Can you work these out from the model? Positions are in its coordinate system, mm. A direction names the side the tool comes from. Give positions to 0.01 mm unless a question says otherwise; leave off trailing zeros. Loops run counter-clockwise (first coordinate to the right, second up) from the corner with the lowest first, then second, coordinate; pieces in that order, holes last. Notation, with made-up numbers: (8, -15.5) -> (50, -15.5) arc R14 ccw to (50, -9.5) -> close; hole circle Ø7 at (37.5, 6.25). An arc over 180 degrees is marked (long way). Use CSV: the item, a comma, the result in double quotes.
from build123d import *

# Parameters (mm, degrees)
F1_DEPTH = 2
F3_DEPTH = 2
F5_DEPTH = 2


with BuildPart() as f1:
    # F0 (on Top) → F1 (new body)
    with BuildSketch(Plane.XY):
        with BuildLine():
            ThreePointArc((49.942072, -2.406128), (49.985516, -1.203413), (50, 0))
            ThreePointArc((50, 0), (49.974201, 1.606012), (49.896829, 3.210366))
            ThreePointArc((49.896829, 3.210366), (43.993208, 6.785947), (48.544998, 11.974273))
            ThreePointArc((48.544998, 11.974273), (47.87884, 14.408911), (47.090663, 16.806829))
            ThreePointArc((47.090663, 16.806829), (40.967156, 18.934106), (43.314795, 24.976559))
            ThreePointArc((43.314795, 24.976559), (41.843566, 27.369983), (40.240229, 29.676994))
            ThreePointArc((40.240229, 29.676994), (33.340682, 29.493226), (34.36487, 36.318806))
            ThreePointArc((34.36487, 36.318806), (32.488197, 38.006802), (30.528729, 39.597938))
            ThreePointArc((30.528729, 39.597938), (24.227214, 38.076901), (22.935377, 44.429365))
            ThreePointArc((22.935377, 44.429365), (20.403718, 45.647435), (17.80764, 46.721386))
            ThreePointArc((17.80764, 46.721386), (12.102725, 42.836614), (9.274139, 49.132376))
            ThreePointArc((9.274139, 49.132376), (6.782782, 49.537802), (4.274139, 49.816982))
            ThreePointArc((4.274139, 49.816982), (-0.204697, 45.130548), (-4.725861, 49.776161))
            ThreePointArc((-4.725861, 49.776161), (-7.514166, 49.432148), (-10.278748, 48.932069))
            ThreePointArc((-10.278748, 48.932069), (-12.977762, 42.57968), (-18.761065, 46.346763))
            ThreePointArc((-18.761065, 46.346763), (-21.076119, 45.3409), (-23.337459, 44.219487))
            ThreePointArc((-23.337459, 44.219487), (-24.571619, 37.855565), (-30.886672, 39.319378))
            ThreePointArc((-30.886672, 39.319378), (-33.046356, 37.522505), (-35.101707, 35.607165))
            ThreePointArc((-35.101707, 35.607165), (-33.937901, 28.803999), (-40.839764, 28.84638))
            ThreePointArc((-40.839764, 28.84638), (-42.243501, 26.748582), (-43.53958, 24.582616))
            ThreePointArc((-43.53958, 24.582616), (-41.137225, 18.561708), (-47.241183, 16.37897))
            ThreePointArc((-47.241183, 16.37897), (-48.086561, 13.69973), (-48.780121, 10.977238))
            ThreePointArc((-48.780121, 10.977238), (-44.122996, 5.883251), (-49.952127, 2.187476))
            ThreePointArc((-49.952127, 2.187476), (-49.99887, -0.336221), (-49.918191, -2.859061))
            ThreePointArc((-49.918191, -2.859061), (-44.642053, -6.62536), (-48.596952, -11.761645))
            ThreePointArc((-48.596952, -11.761645), (-47.859623, -14.472611), (-46.971192, -17.137885))
            ThreePointArc((-46.971192, -17.137885), (-40.299352, -18.905387), (-43.205042, -25.165937))
            ThreePointArc((-43.205042, -25.165937), (-41.879951, -27.314277), (-40.448129, -29.393007))
            ThreePointArc((-40.448129, -29.393007), (-33.973344, -29.708924), (-34.523532, -36.168021))
            ThreePointArc((-34.523532, -36.168021), (-32.437593, -38.050001), (-30.249241, -39.81185))
            ThreePointArc((-30.249241, -39.81185), (-23.680948, -37.691698), (-22.740661, -44.529342))
            ThreePointArc((-22.740661, -44.529342), (-20.464443, -45.620243), (-18.136072, -46.59488))
            ThreePointArc((-18.136072, -46.59488), (-12.518339, -43.360114), (-9.489135, -49.091306))
            ThreePointArc((-9.489135, -49.091306), (-6.716856, -49.546784), (-3.92337, -49.845834))
            ThreePointArc((-3.92337, -49.845834), (0.455989, -44.511162), (4.943718, -49.754996))
            ThreePointArc((4.943718, -49.754996), (7.44838, -49.442104), (9.934059, -49.003209))
            ThreePointArc((9.934059, -49.003209), (12.91115, -43.244774), (18.557995, -46.428448))
            ThreePointArc((18.557995, -46.428448), (21.136435, -45.312814), (23.648143, -44.054118))
            ThreePointArc((23.648143, -44.054118), (24.448153, -37.198646), (31.058502, -39.18379))
            ThreePointArc((31.058502, -39.18379), (32.996395, -37.566446), (34.850197, -35.853364))
            ThreePointArc((34.850197, -35.853364), (34.241441, -29.399524), (40.713093, -29.024886))
            ThreePointArc((40.713093, -29.024886), (42.279058, -26.692345), (43.711539, -24.275531))
            ThreePointArc((43.711539, -24.275531), (40.678202, -18.075823), (47.312431, -16.172008))
            ThreePointArc((47.312431, -16.172008), (48.068288, -13.763707), (48.701644, -11.32033))
            ThreePointArc((48.701644, -11.32033), (44.700316, -6.220133), (49.942072, -2.406128))
        make_face()
    extrude(amount=F1_DEPTH)

    # F2 (on face) → F3 (cut)
    with BuildSketch(Plane.XY.offset(2)):
        with BuildLine():
            Line((8.49059, 0.399851), (9.988929, 0.470413))
            ThreePointArc((9.988929, 0.470413), (9.727268, 2.319537), (9.126347, 4.087762))
            Line((9.126347, 4.087762), (7.738448, 3.516591))
            ThreePointArc((7.738448, 3.516591), (7.46517, 4.064633), (7.153141, 4.591576))
            Line((7.153141, 4.591576), (8.41546, 5.401854))
            ThreePointArc((8.41546, 5.401854), (7.264293, 6.872412), (5.859767, 8.103279))
            Line((5.859767, 8.103279), (4.943397, 6.914682))
            ThreePointArc((4.943397, 6.914682), (4.43271, 7.25266), (3.899014, 7.552992))
            Line((3.899014, 7.552992), (4.587075, 8.885873))
            ThreePointArc((4.587075, 8.885873), (2.854856, 9.58383), (1.023068, 9.947529))
            Line((1.023068, 9.947529), (0.823767, 8.459989))
            ThreePointArc((0.823767, 8.459989), (0.21251, 8.497343), (-0.399851, 8.49059))
            Line((-0.399851, 8.49059), (-0.470413, 9.988929))
            ThreePointArc((-0.470413, 9.988929), (-2.319537, 9.727268), (-4.087762, 9.126347))
            Line((-4.087762, 9.126347), (-3.516591, 7.738448))
            ThreePointArc((-3.516591, 7.738448), (-4.064633, 7.46517), (-4.591576, 7.153141))
            Line((-4.591576, 7.153141), (-5.401854, 8.41546))
            ThreePointArc((-5.401854, 8.41546), (-6.872412, 7.264293), (-8.103279, 5.859767))
            Line((-8.103279, 5.859767), (-6.914682, 4.943397))
            ThreePointArc((-6.914682, 4.943397), (-7.25266, 4.43271), (-7.552992, 3.899014))
            Line((-7.552992, 3.899014), (-8.885873, 4.587075))
            ThreePointArc((-8.885873, 4.587075), (-9.58383, 2.854856), (-9.947529, 1.023068))
            Line((-9.947529, 1.023068), (-8.459989, 0.823767))
            ThreePointArc((-8.459989, 0.823767), (-8.497343, 0.21251), (-8.49059, -0.399851))
            Line((-8.49059, -0.399851), (-9.988929, -0.470413))
            ThreePointArc((-9.988929, -0.470413), (-9.727268, -2.319537), (-9.126347, -4.087762))
            Line((-9.126347, -4.087762), (-7.738448, -3.516591))
            ThreePointArc((-7.738448, -3.516591), (-7.46517, -4.064633), (-7.153141, -4.591576))
            Line((-7.153141, -4.591576), (-8.41546, -5.401854))
            ThreePointArc((-8.41546, -5.401854), (-7.264293, -6.872412), (-5.859767, -8.103279))
            Line((-5.859767, -8.103279), (-4.943397, -6.914682))
            ThreePointArc((-4.943397, -6.914682), (-4.43271, -7.25266), (-3.899014, -7.552992))
            Line((-3.899014, -7.552992), (-4.587075, -8.885873))
            ThreePointArc((-4.587075, -8.885873), (-2.854856, -9.58383), (-1.023068, -9.947529))
            Line((-1.023068, -9.947529), (-0.823767, -8.459989))
            ThreePointArc((-0.823767, -8.459989), (-0.21251, -8.497343), (0.399851, -8.49059))
            Line((0.399851, -8.49059), (0.470413, -9.988929))
            ThreePointArc((0.470413, -9.988929), (2.319537, -9.727268), (4.087762, -9.126347))
            Line((4.087762, -9.126347), (3.516591, -7.738448))
            ThreePointArc((3.516591, -7.738448), (4.064633, -7.46517), (4.591576, -7.153141))
            Line((4.591576, -7.153141), (5.401854, -8.41546))
            ThreePointArc((5.401854, -8.41546), (6.872412, -7.264293), (8.103279, -5.859767))
            Line((8.103279, -5.859767), (6.914682, -4.943397))
            ThreePointArc((6.914682, -4.943397), (7.25266, -4.43271), (7.552992, -3.899014))
            Line((7.552992, -3.899014), (8.885873, -4.587075))
            ThreePointArc((8.885873, -4.587075), (9.58383, -2.854856), (9.947529, -1.023068))
            Line((9.947529, -1.023068), (8.459989, -0.823767))
            ThreePointArc((8.459989, -0.823767), (8.497343, -0.21251), (8.49059, 0.399851))
        make_face()
    extrude(amount=-F3_DEPTH, mode=Mode.SUBTRACT)

    # F4 (on face) → F5 (cut)
    with BuildSketch(Plane.XY.offset(2)):
        with BuildLine():
            ThreePointArc((18.809128, 25.888544), (25.793139, 26.994703), (24.686981, 33.978714))
            ThreePointArc((24.686981, 33.978714), (12.978714, 39.944374), (0, 42))
            ThreePointArc((0, 42), (3.535534, 40.535534), (5, 37))
            ThreePointArc((5, 37), (3.535534, 33.464466), (0, 32))
            ThreePointArc((0, 32), (9.888544, 30.433809), (18.809128, 25.888544))
        make_face()
        with BuildLine():
            ThreePointArc((5, 37), (3.535534, 40.535534), (0, 42))
            ThreePointArc((0, 42), (-5, 37), (0, 32))
            ThreePointArc((0, 32), (3.535534, 33.464466), (5, 37))
        make_face()
        with BuildLine():
            ThreePointArc((-30.433809, 9.888544), (-25.888544, 18.809128), (-18.809128, 25.888544))
            ThreePointArc((-18.809128, 25.888544), (-17.702969, 32.872555), (-24.686981, 33.978714))
            ThreePointArc((-24.686981, 33.978714), (-33.978714, 24.686981), (-39.944374, 12.978714))
            ThreePointArc((-39.944374, 12.978714), (-36.734176, 6.678346), (-30.433809, 9.888544))
        make_face()
        with BuildLine():
            ThreePointArc((-18.809128, -25.888544), (-25.888544, -18.809128), (-30.433809, -9.888544))
            ThreePointArc((-30.433809, -9.888544), (-36.734176, -6.678346), (-39.944374, -12.978714))
            ThreePointArc((-39.944374, -12.978714), (-33.978714, -24.686981), (-24.686981, -33.978714))
            ThreePointArc((-24.686981, -33.978714), (-17.702969, -32.872555), (-18.809128, -25.888544))
        make_face()
        with BuildLine():
            ThreePointArc((18.809128, -25.888544), (9.888544, -30.433809), (0, -32))
            ThreePointArc((0, -32), (-5, -37), (0, -42))
            ThreePointArc((0, -42), (12.978714, -39.944374), (24.686981, -33.978714))
            ThreePointArc((24.686981, -33.978714), (25.793139, -26.994703), (18.809128, -25.888544))
        make_face()
        with BuildLine():
            ThreePointArc((30.433809, 9.888544), (32, 0), (30.433809, -9.888544))
            ThreePointArc((30.433809, -9.888544), (33.644006, -16.188911), (39.944374, -12.978714))
            ThreePointArc((39.944374, -12.978714), (42, 0), (39.944374, 12.978714))
            ThreePointArc((39.944374, 12.978714), (33.644006, 16.188911), (30.433809, 9.888544))
        make_face()
    extrude(amount=-F5_DEPTH, mode=Mode.SUBTRACT)


solid = f1.part
(1) If we section it at B-B, the plane x = -13.5: Write out the boundary of the cut face in (y, z), then the cut area to 3 significant figures.
Answer sheet:
outline,"(-43.19, 0) -> (42.45, 0) -> (42.45, 2) -> (-43.19, 2) -> close"
area,"171 mm2"
(2) If I drill on L1, parallel to Y at x = -19.5, z = 1.5; L2, parallel to Y at x = -20, z = 1.05; L3, parallel to X at y = 5.5, z = 0.5, over which ranges is the centre line in solid material (lowest first)? Write a range as from..to.
Answer sheet:
L1,"y = -46.04..-34.4, -25.37..25.37, 34.4..46.04"
L2,"y = -45.83..-34.62, -24.98..24.98, 34.62..45.83"
L3,"x = -44.19..-7.64, 8.35..31.52, 41.64..44.4"
(3) If we section it at A-A, the plane z = 0.85: Give the number of separate pieces and of enclosed holes in the cut face, then the cut area to 3 significant figures.
Answer sheet:
separate pieces,"1"
enclosed holes,"6"
area,"5,190 mm2"
(4) Will these pins go through, and if not, where does the flat tip stop? pin 1 Ø5.5 at (x, y) = (-37.37, 31.72) entering from -Z; pin 2 Ø1 at (y, z) = (11, 2) entering from -X; pin 3 Ø1 at (x, z) = (-13, 1) entering from -Y.
Answer sheet:
pin 1,"passes through"
pin 2,"stops at x = -48.78"
pin 3,"stops at y = -43.37"
(5) We'd pull the mould along Y, two halves only. Please class faces 1 (the face through (10.02, -30.39, 1.01)), 2 (the face through (42.258, -26.726, 0.986)), 3 (the face through (41.865, 27.337, 0.986)): released by +Y, released by -Y, zero draft, split by the parting line, or undercut.
Answer sheet:
face 1,"undercut"
face 2,"released by -Y"
face 3,"released by +Y"
(6) Which directions (+Z, -Z, +X, -X, +Y, -Y) give clear straight access to the entire face, cutting with the end or side of a thin tool? Please do faces 4 (the face through (-33.87, 24.836, 1.014)), 5 (the face through (-21.044, 45.356, 0.986)).
Answer sheet:
face 4,"+Z, -Z"
face 5,"+Z, -Z, -X, +Y"
